Input: dimensioned drawing with shaded views. Units: mm. Origin: part minimum x, y, z. Coordinates: 2 decimals unless noted, no trailing zeros. Order: outer loops, then holes, each group sorted by start corner. A loop starts at its lowest first (then second) coordinate and runs counter-clockwise, first axis right, second up. Notation, with made-up numbers: (2.25, 55) - (43.25, 55) arc R21 ccw to (43.25, 60) - close; hole circle Ø1 at (83.5, -13.75). An arc over 180 degrees is marked (long way). Answer as CSV lines item,"result". Start each with the question number.
Item 1: First-contact query: pin 1 (10 mm diameter, centred on x = 75, z = 11.5, fed in from -Y); pin 2 (1.5 mm diameter, centred on y = 2, z = 1, fed in from +X); pin 3 (1 mm diameter, centred on x = 77, y = 2, fed in from +Z); pin 4 (0.9 mm diameter, centred on x = 81, y = 1, fed in from -Z). Flat tips, straight axial feed; report the tip coordinate or a pass-through.
Item 2: Section D-D (z = 13). Output: boundary loops of the cut face in (x, y) (1 decimal), and give its area (3 significant figures).
Item 3: Section B-B (y = 0.7). Output: boundary loops of the cut face in (x, z).
Item 4: Section A-A (z = 18). Output: boundary loops of the cut face in (x, y).
Item 5: Material intervals for line 1 along X through (y, z) = (1.45, 23.5) (1 decimal); line 2 along Z through (x, y) = (32.3, 0.6); line 3 along X through (y, z) = (2.85, 15) (1 decimal), sorted ascending.
Item 6: Section C-C (x = 57.7). Output: boundary loops of the cut face in (y, z), and give its area (3 significant figures).
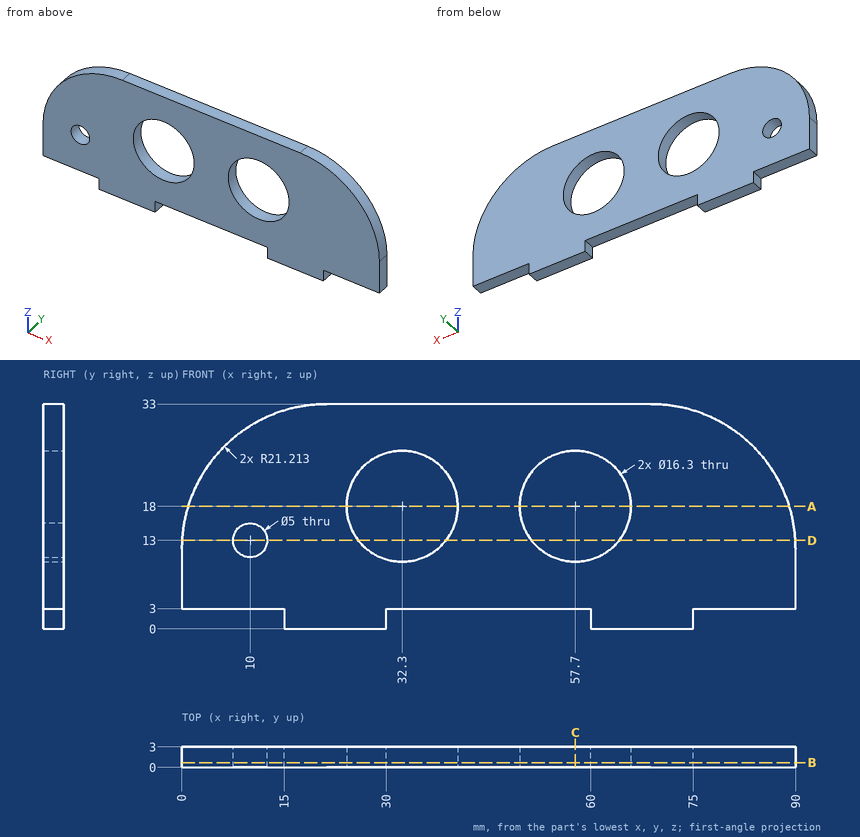
Determined:
1,pin 1,"stops at y = 0"
1,pin 2,"stops at x = 75"
1,pin 3,"stops at z = 31.55"
1,pin 4,"stops at z = 3"
2,outline,"(0, 0) - (7.5, 0) - (7.5, 3) - (0, 3) - close; (12.5, 0) - (25.9, 0) - (25.9, 3) - (12.5, 3) - close; (38.7, 0) - (51.3, 0) - (51.3, 3) - (38.7, 3) - close; (64.1, 0) - (90, 0) - (90, 3) - (64.1, 3) - close"
2,area,"178 mm^2"
3,outline,"(0, 3) - (15, 3) - (15, 0) - (30, 0) - (30, 3) - (60, 3) - (60, 0) - (75, 0) - (75, 3) - (90, 3) - (90, 11.79) arc R21.21 ccw to (68.79, 33) - (21.21, 33) arc R21.21 ccw to (0, 11.79) - close; hole circle Ø5 at (10, 13); hole circle Ø16.3 at (32.3, 18); hole circle Ø16.3 at (57.7, 18)"
4,outline,"(0.93, 0) - (24.15, 0) - (24.15, 3) - (0.93, 3) - close; (40.45, 0) - (49.55, 0) - (49.55, 3) - (40.45, 3) - close; (65.85, 0) - (89.07, 0) - (89.07, 3) - (65.85, 3) - close"
5,line 1,"x = 3.5 to 26.3, 38.3 to 51.7, 63.7 to 86.5"
5,line 2,"z = 3 to 9.85, 26.15 to 33"
5,line 3,"x = 0.2 to 8.5, 11.5 to 24.7, 39.9 to 50.1, 65.3 to 89.8"
6,outline,"(0, 3) - (3, 3) - (3, 9.85) - (0, 9.85) - close; (0, 26.15) - (3, 26.15) - (3, 33) - (0, 33) - close"
6,area,"41.1 mm^2"
